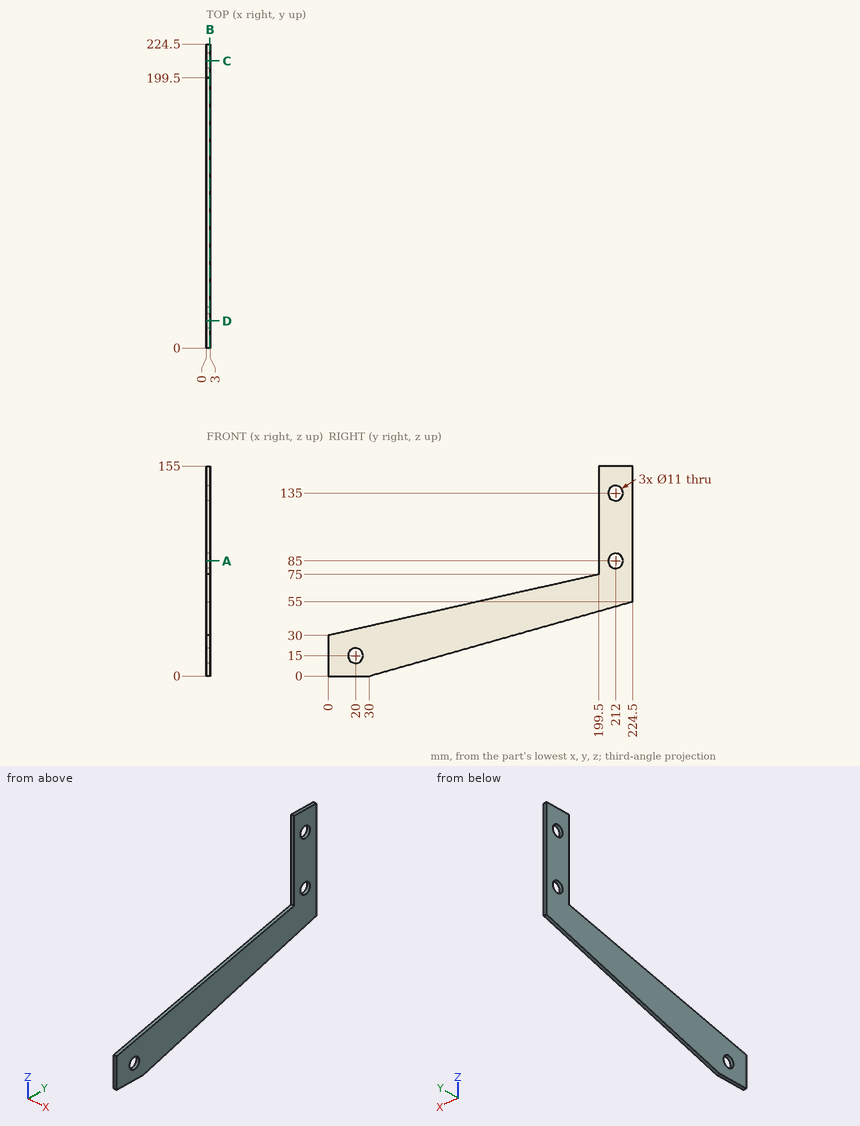
Print and shaded views of the part. All mm, measured from the part's lowest x, y and z. Coordinates: 2 decimals unless noted, no trailing zeros. Write each loop counter-clockwise with the first axis right and the second up, starting at its lowest first coordinate (ties: lowest second). Pieces come first, ordered by that corner, then holes. Notation, with made-up numbers: (9.25, 8) - (45.25, 8) arc R16 ccw to (45.25, 34) - close; hole circle Ø11 at (43.25, 68). An arc over 180 degrees is marked (long way). One line per question, with ' | ' between items. Start each with the question number.
Q1. Drill centre lines: line 1 (Z direction, x = 1.4, y = 208); line 2 (Z direction, x = 0.7, y = 207); line 3 (Y direction, x = 2.45, z = 118.5). Where is each one in solid material? Low to high. Write a range as [from, to].
Q2. Cut at A-A, the plane z = 85. List the corners of the cut face in (x, y).
Q3. Cut at C-C, the plane y = 212. List the corners of the cut face in (x, z), then the cut area to 3 significant figures.
Q4. Pin check, flat tips, straight feed: pin 1 (10 mm diameter, centred on y = 20, z = 15, fed in from +X); pin 2 (1.5 mm diameter, centred on x = 1, y = 187, fed in from +Z). Stop position of each tip, or through.
Q5. Cut at D-D, the plane y = 20. List the corners of the cut face in (x, z).
Q6. Cut at B-B, the plane x = 2.5. List the corners of the cut face in (y, z), then the cut area to 3 significant figures.
Answer below:
1) line 1: [50.33, 81.23], [88.77, 131.23], [138.77, 155] | line 2: [50.05, 82.71], [87.29, 132.71], [137.29, 155] | line 3: [199.5, 224.5]
2) outline: (0, 199.5) - (3, 199.5) - (3, 206.5) - (0, 206.5) - close; (0, 217.5) - (3, 217.5) - (3, 224.5) - (0, 224.5) - close
3) outline: (0, 51.47) - (3, 51.47) - (3, 79.5) - (0, 79.5) - close; (0, 90.5) - (3, 90.5) - (3, 129.5) - (0, 129.5) - close; (0, 140.5) - (3, 140.5) - (3, 155) - (0, 155) - close | area: 245 mm^2
4) pin 1: through | pin 2: z = 72.35
5) outline: (0, 0) - (3, 0) - (3, 9.5) - (0, 9.5) - close; (0, 20.5) - (3, 20.5) - (3, 34.51) - (0, 34.51) - close
6) outline: (0, 0) - (30, 0) - (224.5, 55) - (224.5, 155) - (199.5, 155) - (199.5, 75) - (0, 30) - close; hole circle Ø11 at (20, 15); hole circle Ø11 at (212, 85); hole circle Ø11 at (212, 135) | area: 8,710 mm^2
